from build123d import *

# Parameters (mm, degrees)
UPN_UPN180_1_DEPTH = 700
SKETCH128_R        = 15
CUT_EXTRUDE1_DEPTH = 10
FILLET1_R          = 2


with BuildPart() as part:
    # Sketch133 → Upn UPN180(1) (new body)
    with BuildSketch(Plane.ZX.offset(-309.124087591)):
        with BuildLine():
            Line((70, 180), (0, 180))
            Line((0, 180), (0, 0))
            Line((0, 0), (70, 0))
            Line((70, 0), (70, 3.122386663))
            ThreePointArc((70, 3.122386663), (68.541183887, 6.853181859), (64.938606257, 8.604870092))
            Line((64.938606257, 8.604870092), (18.122787486, 12.350200343))
            ThreePointArc((18.122787486, 12.350200343), (10.917632226, 15.85357681), (8, 23.315167202))
            Line((8, 23.315167202), (8, 156.684832798))
            ThreePointArc((8, 156.684832798), (10.917632226, 164.14642319), (18.122787486, 167.649799657))
            Line((18.122787486, 167.649799657), (64.938606257, 171.395129908))
            ThreePointArc((64.938606257, 171.395129908), (68.541183887, 173.146818141), (70, 176.877613337))
            Line((70, 176.877613337), (70, 180))
        make_face()
    extrude(amount=UPN_UPN180_1_DEPTH)

    # Sketch128 → Cut-Extrude1 (cut)
    with BuildSketch(Plane.XY.offset(8)):
        with Locations((90, 280.875912409)):
            Circle(SKETCH128_R)
    extrude(amount=-CUT_EXTRUDE1_DEPTH, mode=Mode.SUBTRACT)

    # Fillet1
    fillet1_edges = [part.edges().sort_by_distance(p)[0] for p in [
        (169.522464782, -309.124087591, 41.530696872),
        (164.14642319, -309.124087591, 10.917632226),
        (180, 390.875912409, 35),
        (90, -309.124087591, 8),
        (15.85357681, -309.124087591, 10.917632226),
        (10.477535218, -309.124087591, 41.530696872),
        (6.853181859, -309.124087591, 68.541183887),
        (1.561193332, -309.124087591, 70),
        (0, -309.124087591, 35),
        (90, -309.124087591, 0),
        (180, -309.124087591, 35),
        (178.438806668, -309.124087591, 70),
        (173.146818141, -309.124087591, 68.541183887),
        (90, 390.875912409, 0),
        (0, 390.875912409, 35),
        (0, 40.875912409, 70),
        (0, 40.875912409, 0),
        (180, 40.875912409, 0),
        (180, 40.875912409, 70),
        (1.561193332, 390.875912409, 70),
        (6.853181859, 390.875912409, 68.541183887),
        (10.477535218, 390.875912409, 41.530696872),
        (15.85357681, 390.875912409, 10.917632226),
        (90, 390.875912409, 8),
        (164.14642319, 390.875912409, 10.917632226),
        (169.522464782, 390.875912409, 41.530696872),
        (173.146818141, 390.875912409, 68.541183887),
        (178.438806668, 390.875912409, 70),
    ]]
    fillet(fillet1_edges, radius=FILLET1_R)


solid = part.part
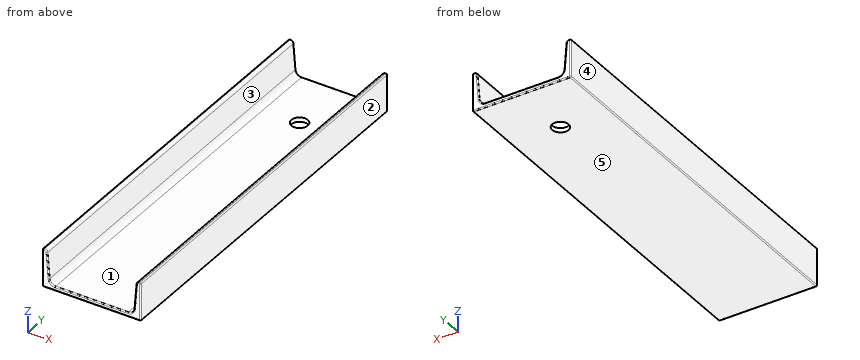
Design review of the part built by this model. Coordinates are the model's own, in mm. Face numbers are marked on the shaded views. A direction names the side the tool comes from. Round coordinates to 2 decimals unless told otherwise and drop trailing zeros. Write each loop counter-clockwise with the first axis right and the second up, starting at its lowest first coordinate (ties: lowest second). Pieces come first, ordered by that corner, then holes. Notation, with made-up numbers: M 11.5,78 L 56.5,78 A29 ccw 56.5,108 Z; hole C -2,29 d2. An arc over 180 degrees is marked long. One line per item, written item: value. Start each with the question number.
1. Clearance check with flat-ended pins moving along their axes: P1, Ø10, axis at x = 139, y = -214.5, coming from the +Z side; P2, Ø8, axis at x = 100.5, z = 9, coming from the +Y side. State where each tip first meets the part, or that it passes through.
2. To check wall thickness, follow probe 1 along Y at (x, z) = (90, 2.25); probe 2 along X at (y, z) = (-130, 43.5); probe 3 along Z at (x, y) = (27, 305). State the ranges of each line that lie inside material, in increasing order. Write a range as from..to.
3. Take a section at A-A on x = 90. State the section outline as (y, z) points.
4. For the marked faces 1 and 2, list the 3-axis set-ups (+Z, -Z, +X, -X, +Y, -Y) from which the entire face can be reached by the end or side of a thin tool; tool diameter is ignored.
5. Take a section at C-C on x = 139. State the section outline as (y, z) points.
6. Take a section at B-B on y = 314. State the section outline as (x, z) points, then the cut area to 3 significant figures.
7. Draft analysis for pull direction X (two halves, no side actions). For the marked faces 3, 4 and 5, state which applies: pulls with the +X half, pulls with the -X half, needs draft (parallel to the pull), parting line crosses it, or undercut.
Computed:
1. P1: stops at z = 8
1. P2: stops at y = 390.88
2. probe 1: y = -309.12..265.88, 295.88..390.88
2. probe 2: x = 0..10.32, 169.68..180
2. probe 3: z = 0..8
3. outline: M -309.12,2 A2 ccw -307.12,0 L 265.88,0 L 265.88,8 L -307.12,8 A2 ccw -309.12,6 Z; M 295.88,0 L 388.88,0 A2 ccw 390.88,2 L 390.88,6 A2 ccw 388.88,8 L 295.88,8 Z
4. face 1: +Z, +Y, -Y
4. face 2: +Z, -Z, +X, +Y, -Y
5. outline: M -309.12,2 A2 ccw -307.12,0 L 388.88,0 A2 ccw 390.88,2 L 390.88,6 A2 ccw 388.88,8 L -307.12,8 A2 ccw -309.12,6 Z
6. outline: M 0,2 A2 ccw 2,0 L 178,0 A2 ccw 180,2 L 180,68 A2 ccw 178,70 L 176.88,70 A5.5 ccw 171.4,64.94 L 167.65,18.12 A11 cw 156.68,8 L 23.32,8 A11 cw 12.35,18.12 L 8.6,64.94 A5.5 ccw 3.12,70 L 2,70 A2 ccw 0,68 Z
6. area: 2,790 mm²
7. face 3: undercut
7. face 4: pulls with the -X half
7. face 5: needs draft
